```python
from build123d import *

# Parameters (mm, degrees)
SKETCH1_W           = 5.33
SKETCH1_H           = 4.06
BASE_EXTRUDE_DEPTH  = 3.81
SKETCH2_R           = 0.35
BOSS_EXTRUDE1_DEPTH = 3
DOME1_FACE_RADIUS   = 0.35
DOME1_HEIGHT        = 0.35
DOME2_FACE_RADIUS   = 0.35
DOME2_HEIGHT        = 0.35


with BuildPart() as part:
    # Sketch1 → Base-Extrude (new body)
    with BuildSketch(Plane(origin=(0, 0, 0), x_dir=(1, 0, 0), z_dir=(0, 1, 0))):
        with Locations((-1.265, 0)):
            Rectangle(SKETCH1_W, SKETCH1_H)
    extrude(amount=BASE_EXTRUDE_DEPTH)

    # Sketch2 → Boss-Extrude1 (add)
    with BuildSketch(Plane.XZ):
        Circle(SKETCH2_R)
        with Locations((-2.53, 0)):
            Circle(SKETCH2_R)
    extrude(amount=BOSS_EXTRUDE1_DEPTH)

    # Dome1: a dome of height H over a round flat face of radius A is a cap of a sphere of radius (A * A + H * H) / (2 * H)
    dome1_r = (DOME1_FACE_RADIUS * DOME1_FACE_RADIUS + DOME1_HEIGHT * DOME1_HEIGHT) / (2 * DOME1_HEIGHT)
    dome1_base = Plane((0, -3, 0), z_dir=(0, -1, 0))
    with Locations(dome1_base.offset(DOME1_HEIGHT - dome1_r)):
        dome1_ball = Sphere(dome1_r, mode=Mode.PRIVATE)
    add(split(dome1_ball, bisect_by=dome1_base, keep=Keep.TOP, mode=Mode.PRIVATE))

    # Dome2: a dome of height H over a round flat face of radius A is a cap of a sphere of radius (A * A + H * H) / (2 * H)
    dome2_r = (DOME2_FACE_RADIUS * DOME2_FACE_RADIUS + DOME2_HEIGHT * DOME2_HEIGHT) / (2 * DOME2_HEIGHT)
    dome2_base = Plane((-2.53, -3, 0), z_dir=(0, -1, 0))
    with Locations(dome2_base.offset(DOME2_HEIGHT - dome2_r)):
        dome2_ball = Sphere(dome2_r, mode=Mode.PRIVATE)
    add(split(dome2_ball, bisect_by=dome2_base, keep=Keep.TOP, mode=Mode.PRIVATE))


solid = part.part
```
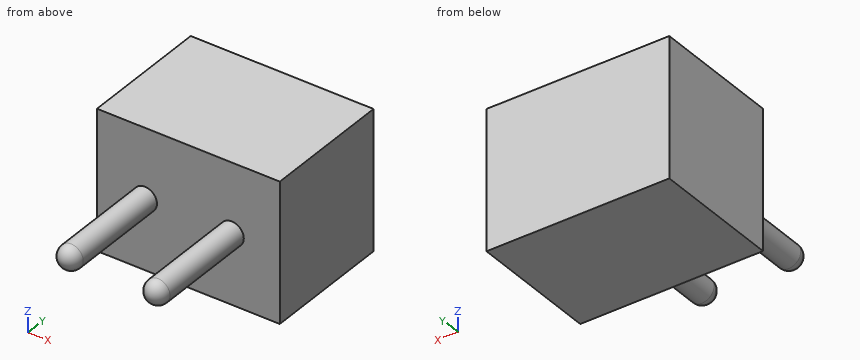
Geometry check sheet. Reference: the model listing, model coordinates, mm. Give positions to 0.01 mm unless a question says otherwise; leave off trailing zeros. Order: outer loops, then holes, each group sorted by start corner. A loop starts at its lowest first (then second) coordinate and runs counter-clockwise, first axis right, second up.
1. Gauge pin test, flat end, axial feed: pin 1 Ø1.2 at (x, z) = (-1, -0.5) entering from -Y. Record the tip position at first contact, or that the pin passes through.
2. Section check C-C, the plane x = -2.53. Enter the section's corners in (y, z).
3. Section check B-B, the plane z = 0. Enter the section's corners in (x, y).
4. Thickness scan on L1, parallel to Y at x = -1.55, z = 1.45; L2, parallel to Z at x = -0.25, y = -2. Record the ranges inside material, lowest first.
5. Section check D-D, the plane z = 0.65. Enter the section's corners in (x, y), and give its area (3 significant figures).
6. Section check A-A, the plane y = -2.25. Enter the section's corners in (x, z), and give its area (3 significant figures).
Values follow:
1. pin 1: stops at y = 0
2. outline: (-3, -0.35) - (0, -0.35) - (0, -2.03) - (3.81, -2.03) - (3.81, 2.03) - (0, 2.03) - (0, 0.35) - (-3, 0.35) arc R0.35 ccw to start
3. outline: (-3.93, 0) - (-2.88, 0) - (-2.88, -3) arc R0.35 ccw to (-2.18, -3) - (-2.18, 0) - (-0.35, 0) - (-0.35, -3) arc R0.35 ccw to (0.35, -3) - (0.35, 0) - (1.4, 0) - (1.4, 3.81) - (-3.93, 3.81) - close
4. L1: y = 0 to 3.81
4. L2: z = -0.24 to 0.24
5. outline: (-3.93, 0) - (1.4, 0) - (1.4, 3.81) - (-3.93, 3.81) - close
5. area: 20.3 mm2
6. outline: circle Ø0.7 at (-2.53, 0); circle Ø0.7 at (0, 0)
6. area: 0.770 mm2
